Could you check a few things on this model? Use its own coordinates, in mm. Give positions to 0.01 mm unless a question says otherwise; leave off trailing zeros. Order: outer loops, then holes, each group sorted by start corner. A loop starts at its lowest first (then second) coordinate and runs counter-clockwise, first axis right, second up. Notation, with made-up numbers: (-14.75, 45.25) -> (-9.75, 45.25) arc R12 cw to (-9.75, 53.25) -> close; hole circle Ø6 at (48.5, 71). An arc over 180 degrees is marked (long way). Answer as CSV lines item,"result". Start each with the question number.
(1) I need wall thicknesses on L1, parallel to X at y = 0.3, z = 2; L2, parallel to Z at x = 38, y = 1.1; L3, parallel to X at y = 0.7, z = 2.45. Which ranges of each line are inside material? Lowest first, please.
(2) I want a section at B-B (x = 50). Please give me the cut outline in (y, z), plus the area to 3 significant figures.
(3) Will this pin go through, and if not, where does the flat tip stop? pin 1 Ø1 at (x, z) = (-40, 2.5) entering from +Y.
(4) I want a section at A-A (x = -12). Please give me the cut outline in (y, z), plus the area to 3 significant figures.
```python
from build123d import *

# Parameters (mm, degrees)
SKICA2_W                = 150
SKICA2_H                = 4.6
SKICA2_W_2              = 18
SKICA2_H_2              = 1
P_IDAT_VYSUNUT_M2_DEPTH = 0.8
SKICA3_R                = 1.75
P_IDAT_VYSUNUT_M3_DEPTH = 2
ZAOBLIT1_R              = 0.5


with BuildPart() as part:
    # Skica2 → Přidat vysunutím2 (new body)
    with BuildSketch(Plane.XY):
        Rectangle(SKICA2_W, SKICA2_H)
        with Locations((-5, 0)):
            Rectangle(SKICA2_W_2, SKICA2_H_2, mode=Mode.SUBTRACT)
    extrude(amount=P_IDAT_VYSUNUT_M2_DEPTH)

    # Skica3 → Přidat vysunutím3 (add)
    with BuildSketch(Plane.XY.offset(0.8)):
        with Locations((-50, 0)):
            Circle(SKICA3_R)
        with Locations((50, 0)):
            Circle(SKICA3_R)
    extrude(amount=P_IDAT_VYSUNUT_M3_DEPTH)

    # Zaoblit1
    zaoblit1_edges = [part.edges().sort_by_distance(p)[0] for p in [
        (-51.75, 0, 2.8),
        (48.25, 0, 2.8),
    ]]
    fillet(zaoblit1_edges, radius=ZAOBLIT1_R)


solid = part.part
```
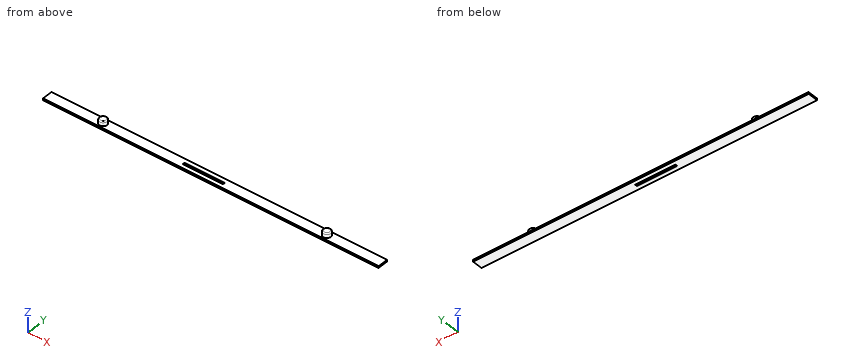
Final values:
1,L1,"-51.72 to -48.28, 48.28 to 51.72"
1,L2,"0 to 0.8"
1,L3,"-51.58 to -48.42, 48.42 to 51.58"
2,outline,"(-2.3, 0) -> (2.3, 0) -> (2.3, 0.8) -> (1.75, 0.8) -> (1.75, 2.3) arc R0.5 ccw to (1.25, 2.8) -> (-1.25, 2.8) arc R0.5 ccw to (-1.75, 2.3) -> (-1.75, 0.8) -> (-2.3, 0.8) -> close"
2,area,"10.6 mm²"
3,pin 1,"through"
4,outline,"(-2.3, 0) -> (-0.5, 0) -> (-0.5, 0.8) -> (-2.3, 0.8) -> close; (0.5, 0) -> (2.3, 0) -> (2.3, 0.8) -> (0.5, 0.8) -> close"
4,area,"2.88 mm²"
